Check sheet for the modelled part. Datum: model origin and axes. Units: mm. Face numbers are marked on the shaded views. Give positions to 0.01 mm unless a question says otherwise; leave off trailing zeros. Loops run counter-clockwise (first coordinate to the right, second up) from the corner with the lowest first, then second, coordinate; pieces in that order, holes last. Notation, with made-up numbers: (55, 25) - (96, 25) arc R25 ccw to (96, 54) - close; hole circle Ø7 at (-15, 72.25). An arc over 180 degrees is marked (long way). Use CSV: the item, a comma, the result in double quotes.
from build123d import *
from OCP.BRepFilletAPI import BRepFilletAPI_MakeChamfer

# Parameters (mm, degrees)
SKETCH1_R           = 50
BOSS_EXTRUDE1_DEPTH = 254.135358
SKETCH2_R           = 27.057401957
CUT_EXTRUDE1_DEPTH  = 264.78927231
CHAMFER1_SIZE       = 3.322504
CHAMFER1_SIZE2      = 2.763299


with BuildPart() as part:
    # Sketch1 → Boss-Extrude1 (new body)
    with BuildSketch(Plane(origin=(0, 0, 0), x_dir=(1, 0, 0), z_dir=(0, 1, 0))):
        with Locations(Location((0, 0, 0), (0, 0, 270))):
            Circle(SKETCH1_R)
    extrude(amount=BOSS_EXTRUDE1_DEPTH)

    # Sketch2 → Cut-Extrude1 (cut, through all)
    with BuildSketch(Plane(origin=(0, 0, 0), x_dir=(1, 0, 0), z_dir=(0, 1, 0))):
        with Locations(Location((0, 0, 0), (0, 0, 270))):
            Circle(SKETCH2_R)
    extrude(amount=CUT_EXTRUDE1_DEPTH, mode=Mode.SUBTRACT)

    # Chamfer1: one chamfer whose edges measure the first distance from different faces: ONE call of the kernel's chamfer builder (chamfer() names one face for all edges)
    chamfer1_edges_1 = [part.edges().sort_by_distance(p)[0] for p in [
        (0, 0, -50),
    ]]
    chamfer1_side_1 = [part.faces().sort_by_distance(p)[0] for p in [
        (0, 0, -48.585786438),
    ]]
    chamfer1_edges_2 = [part.edges().sort_by_distance(p)[0] for p in [
        (0, 254.135358, -50),
    ]]
    chamfer1_side_2 = [part.faces().sort_by_distance(p)[0] for p in [
        (0, 127.067679, -50),
    ]]
    chamfer1_edges_3 = [part.edges().sort_by_distance(p)[0] for p in [
        (0, 0, -27.057401957),
    ]]
    chamfer1_side_3 = [part.faces().sort_by_distance(p)[0] for p in [
        (0, 127.067679, -27.057401957),
    ]]
    chamfer1_edges_4 = [part.edges().sort_by_distance(p)[0] for p in [
        (0, 254.135358, -27.057401957),
    ]]
    chamfer1_side_4 = [part.faces().sort_by_distance(p)[0] for p in [
        (0, 254.135358, -48.585786438),
    ]]
    chamfer1 = BRepFilletAPI_MakeChamfer(part.part.solid().wrapped)
    for e in chamfer1_edges_1:
        chamfer1.Add(CHAMFER1_SIZE, CHAMFER1_SIZE2, e.wrapped, chamfer1_side_1[0].wrapped)  # the first distance lies on this face
    for e in chamfer1_edges_2:
        chamfer1.Add(CHAMFER1_SIZE, CHAMFER1_SIZE2, e.wrapped, chamfer1_side_2[0].wrapped)  # the first distance lies on this face
    for e in chamfer1_edges_3:
        chamfer1.Add(CHAMFER1_SIZE, CHAMFER1_SIZE2, e.wrapped, chamfer1_side_3[0].wrapped)  # the first distance lies on this face
    for e in chamfer1_edges_4:
        chamfer1.Add(CHAMFER1_SIZE, CHAMFER1_SIZE2, e.wrapped, chamfer1_side_4[0].wrapped)  # the first distance lies on this face
    add(Compound.cast(chamfer1.Shape()), mode=Mode.REPLACE)


solid = part.part
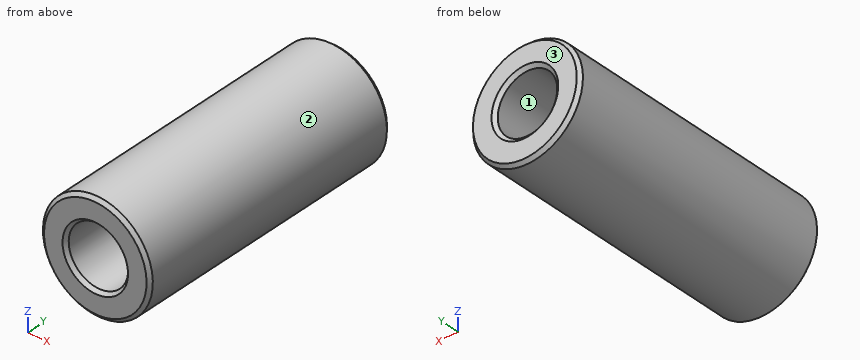
1. Sectioned sample at A-A, the plane x = 0. Record the boundary of the cut face in (y, z).
Completed:
outline,"(0, -46.68) - (2.76, -50) - (250.81, -50) - (254.14, -47.24) - (254.14, -30.38) - (251.37, -27.06) - (3.32, -27.06) - (0, -29.82) - close; (0, 29.82) - (3.32, 27.06) - (251.37, 27.06) - (254.14, 30.38) - (254.14, 47.24) - (250.81, 50) - (2.76, 50) - (0, 46.68) - close"
2. Scan lines: line 1 along X through (y, z) = (153, 0); line 2 along Z through (x, y) = (0.5, 215); line 3 along Z through (x, y) = (-18, 48). Record each from-to range of solid material in increasing order.
Completed:
line 1,"x = -50 to -27.06, 27.06 to 50"
line 2,"z = -50 to -27.05, 27.05 to 50"
line 3,"z = -46.65 to -20.2, 20.2 to 46.65"
3. Go/stop test with flat-tipped pins: pin 1 Ø3 at (x, y) = (24.5, 33) entering from -Z; pin 2 Ø1 at (x, y) = (24, 28) entering from -Z; pin 3 Ø2 at (y, z) = (151, 34) entering from -X. Record where each tip stops, or that it passes through.
Completed:
pin 1,"stops at z = -44.4"
pin 2,"stops at z = -44.13"
pin 3,"stops at x = -37.56"
4. Release check for a two-part mould opening along Z. For the marked faces 1, 2 and 3 record: released by +Z, released by -Z, zero draft, split by the parting line, or undercut.
Completed:
face 1,"undercut"
face 2,"split by the parting line"
face 3,"zero draft"
5. Sectioned sample at B-B, the plane z = 0. Record the boundary of the cut face in (x, y), and give its area (3 significant figures).
Completed:
outline,"(-50, 2.76) - (-46.68, 0) - (-29.82, 0) - (-27.06, 3.32) - (-27.06, 251.37) - (-30.38, 254.14) - (-47.24, 254.14) - (-50, 250.81) - close; (27.06, 3.32) - (29.82, 0) - (46.68, 0) - (50, 2.76) - (50, 250.81) - (47.24, 254.14) - (30.38, 254.14) - (27.06, 251.37) - close"
area,"11,600 mm²"
6. Sectioned sample at C-C, the plane y = 22. Record the boundary of the cut face in (x, z), and give its area (3 significant figures).
Completed:
outline,"circle Ø100 at (0, 0); hole circle Ø54.11 at (0, 0)"
area,"5,550 mm²"
